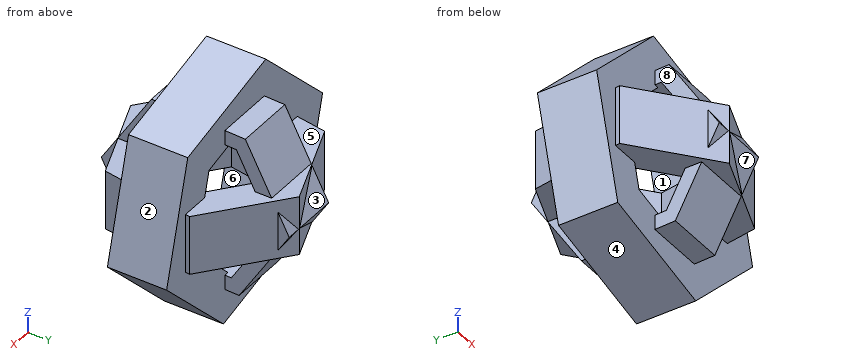
```python
from build123d import *

# Parameters (mm, degrees)
F1_DEPTH = 12.7
F3_DEPTH = 12.7
F5_DEPTH = 12.7


with BuildPart() as f1:
    # F0 (on Top) → F1 (new body, symmetric)
    with BuildSketch(Plane.XY):
        Polygon((-38.285638, -14.609469), (-6.490647, -40.46107), (31.79499, -25.8516), (38.285638, 14.609469), (6.490647, 40.46107), (-31.79499, 25.8516), align=None)
        Polygon((20.380874, -16.571108), (-4.160563, -25.935908), (-24.541437, -9.364801), (-20.380874, 16.571108), (4.160563, 25.935908), (24.541437, 9.364801), align=None, mode=Mode.SUBTRACT)
    extrude(amount=F1_DEPTH, both=True)

    # F2 (on Front) → F3 (join, symmetric)
    with BuildSketch(Plane.XZ):
        Polygon((-36.587807, -36.830874), (13.602569, -50.101408), (50.190376, -13.270534), (36.587807, 36.830874), (-13.602569, 50.101408), (-50.190376, 13.270534), align=None)
        Polygon((31.404369, -8.303439), (8.511195, -31.348701), (-22.893174, -23.045262), (-31.404369, 8.303439), (-8.511195, 31.348701), (22.893174, 23.045262), align=None, mode=Mode.SUBTRACT)
    extrude(amount=F3_DEPTH, both=True)

    # F4 (on Right) → F5 (join, symmetric)
    with BuildSketch(Plane.YZ):
        Polygon((-18.805379, 35.656759), (-40.282349, 1.542443), (-21.47697, -34.114316), (18.805379, -35.656759), (40.282349, -1.542443), (21.47697, 34.114316), align=None)
        Polygon((-17.626668, -27.998443), (-33.060696, 1.265921), (-15.434029, 29.264363), (17.626668, 27.998443), (33.060696, -1.265921), (15.434029, -29.264363), align=None, mode=Mode.SUBTRACT)
    extrude(amount=F5_DEPTH, both=True)


solid = f1.part
```
Work out the finished part from the listing and answer in its coordinate system (mm). Face numbers are marked on the shaded views. A direction names the side the tool comes from. Coordinates: 2 decimals unless noted, no trailing zeros. Loops run counter-clockwise (first coordinate to the right, second up) from the corner with the lowest first, then second, coordinate; pieces in that order, holes last.
1) Section C-C (z = 31) is taken. Give the vertices of the cut face in (x, y).
Results:
outline: (-32.58, -12.7) - (-12.7, -12.7) - (-12.7, -21.74) - (12.7, -21.74) - (12.7, -12.7) - (38.17, -12.7) - (38.17, 12.7) - (12.7, 12.7) - (12.7, 23.12) - (-12.7, 23.12) - (-12.7, 12.7) - (-32.58, 12.7) - close
2) For the marked faces 5, 6, 7 and 8, determine the directions among +Z, -Z, +X, -X, +Y, -Y from which every point of the face is accessible in a straight line to the end or side of a thin tool.
Results:
face 5: none
face 6: +Y, -Y
face 7: -Z, +X, -Y
face 8: +Z, -X, -Y
3) Section D-D (x = -30) is taken. Give the vertices of the cut face in (y, z), plus the area to 3 significant figures.
Results:
outline: (-21.35, -12.7) - (-12.7, -12.7) - (-12.7, -38.57) - (12.7, -38.57) - (12.7, -12.7) - (26.54, -12.7) - (26.54, 12.7) - (12.7, 12.7) - (12.7, 33.6) - (-12.7, 33.6) - (-12.7, 12.7) - (-21.35, 12.7) - close
area: 2,400 mm2
4) Section B-B (y = -6.5) is taken. Give the vertices of the cut face in (x, z).
Results:
outline: (-50.19, 13.27) - (-36.59, -36.83) - (13.6, -50.1) - (50.19, -13.27) - (36.59, 36.83) - (-13.6, 50.1) - close; hole (-27.04, 12.7) - (-24.08, 12.7) - (-24.08, -12.7) - (-25.7, -12.7) - (-22.89, -23.05) - (-2.55, -28.42) - (11.42, -28.42) - (27.04, -12.7) - (22, -12.7) - (22, 12.7) - (25.7, 12.7) - (22.89, 23.05) - (0.67, 28.92) - (-10.92, 28.92) - close
5) Flat-ended cylindrical pins translate along their axes: pin 1 (1 mm diameter, centred on x = 1.5, y = 29.5, fed in from +Z); pin 2 (4 mm diameter, centred on x = -31.5, z = -36.5, fed in from +Y); pin 3 (2 mm diameter, centred on x = -38, z = -19, fed in from -Y). Find the tip coordinate at first contact, or state that the pin passes through.
Results:
pin 1: stops at z = 19.85
pin 2: stops at y = 12.7
pin 3: stops at y = -12.7
6) For a pull along X with two mould halves and no side action, classify the marked faces 1, 2, 3 and 4 as +X half, -X half, draft (parallel to the pull), parting line (faces both ways), or undercut.
Results:
face 1: undercut
face 2: +X half
face 3: draft
face 4: -X half
7) Section A-A (x = -17) is taken. Give the vertices of the cut face in (y, z), plus the area to 3 significant figures.
Results:
outline: (-31.92, -12.7) - (-15.5, -12.7) - (-15.5, 12.7) - (-31.92, 12.7) - close; (-12.7, -42.01) - (12.7, -42.01) - (12.7, -24.6) - (-12.7, -24.6) - close; (-12.7, 22.8) - (12.7, 22.8) - (12.7, 46.68) - (-12.7, 46.68) - close; (17.86, -12.7) - (31.5, -12.7) - (31.5, 12.7) - (17.86, 12.7) - close
area: 1,810 mm2
8) Consider probe 1 along X at (y, z) = (-19, -32). Determine where the line is inside the solid, lowest interval first.
Results:
probe 1: x = -12.7 to 12.7
